The figure shows three views and two pictorial views of one solid part (mm, origin at its lowest corner). Answer the questions. A direction names the side the tool comes from. Coordinates: 2 decimals unless noted, no trailing zeros. Loops run counter-clockwise (first coordinate to the right, second up) from the corner with the lowest first, then second, coordinate; pieces in that order, holes last. Notation, with made-up numbers: M 55.25,47 L 111.25,47 A23 ccw 111.25,60 Z; hole C 77,-25 d4. An arc over 180 degrees is marked long. Return JSON: item names as keys, results as strings. Group by question number.
1. Straight lines are drawn through the part: L1, parallel to X at y = 7.5, z = 41.5; L2, parallel to Z at x = 100, y = 7.7. For each, find the intervals that lie inside material, in ascending order. Write a range as from..to.
2. Section B-B (x = 100) is taken. Write down the section's boundary in (y, z), then the cut area to 3 significant figures.
3. Which of the six approach directions +Z, -Z, +X, -X, +Y, -Y give full straight-line access (tool end or side, diameter ignored) to the marked faces 3 and 4?
4. Section A-A (x = 55) is taken. Write down the section's boundary in (y, z), then the cut area to 3 significant figures.
5. Section D-D (z = 100) is taken. Write down the section's boundary in (x, y).
6. The mould has two halves that part along X. Classify the marked faces 1 and 2: pulls with the +X half, pulls with the -X half, needs draft (parallel to the pull), parting line crosses it, or undercut.
7. Section C-C (y = 8.75) is taken. Write down the section's boundary in (x, z), then the cut area to 3 significant figures.
8. Given P1, Ø4, axis at x = 10, z = 55, coming from the -Y side; P2, Ø1.5, axis at x = 41, z = 75, coming from the -Y side; P3, Ø6, axis at y = 5, z = 16.5, coming from the +X side; P4, Ø5, axis at x = 39, y = 6.5, coming from the -Z side, each flat-ended and moving along its own axis, determine where each tip first touches the part or whether it passes through.
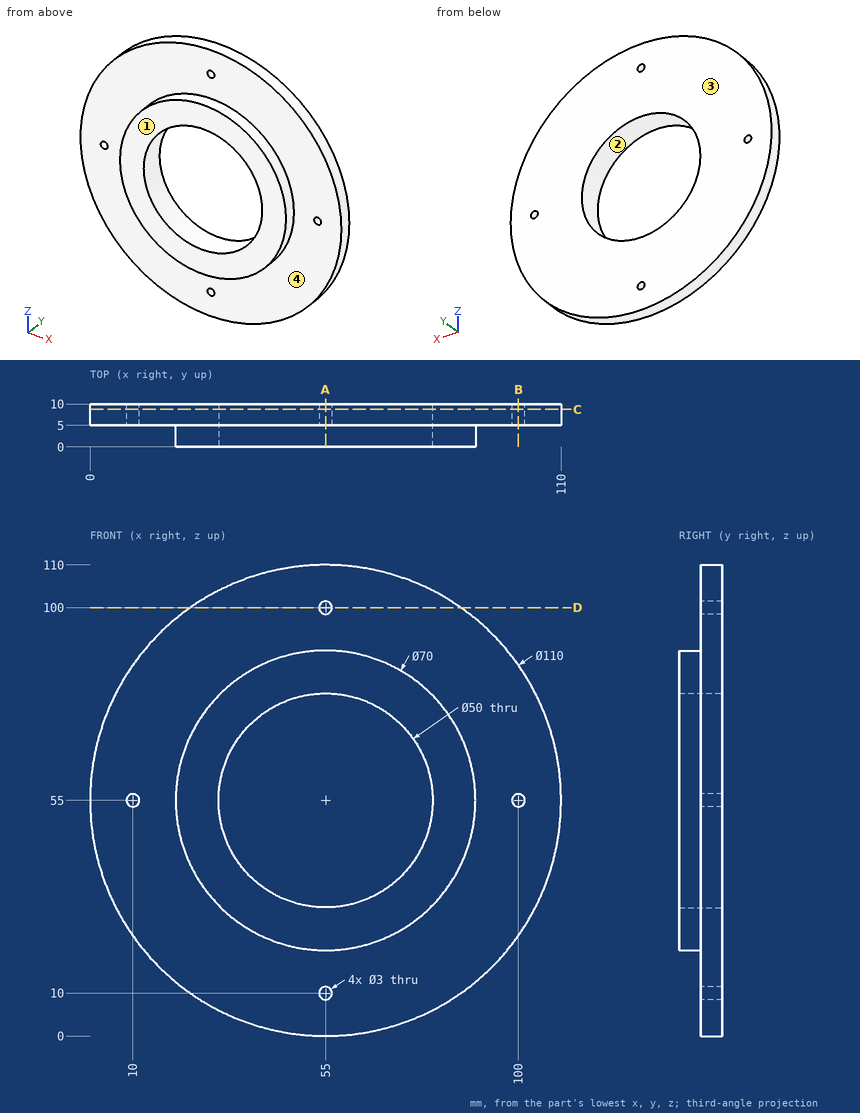
Worked out:
{
 "1": {"L1": "1.68..33.96, 76.04..108.32", "L2": "23.38..53.5, 56.5..86.62"},
 "2": {"outline": "M 5,23.38 L 10,23.38 L 10,53.5 L 5,53.5 Z; M 5,56.5 L 10,56.5 L 10,86.62 L 5,86.62 Z", "area": "301 mm^2"},
 "3": {"face 3": "+Z, -Z, +X, -X, +Y", "face 4": "-Y"},
 "4": {"outline": "M 0,20 L 5,20 L 5,11.5 L 10,11.5 L 10,30 L 0,30 Z; M 0,80 L 10,80 L 10,98.5 L 5,98.5 L 5,90 L 0,90 Z; M 5,0 L 10,0 L 10,8.5 L 5,8.5 Z; M 5,101.5 L 10,101.5 L 10,110 L 5,110 Z", "area": "370 mm^2"},
 "5": {"outline": "M 23.38,5 L 53.5,5 L 53.5,10 L 23.38,10 Z; M 56.5,5 L 86.62,5 L 86.62,10 L 56.5,10 Z"},
 "6": {"face 1": "needs draft", "face 2": "undercut"},
 "7": {"outline": "C 55,55 d110; hole C 10,55 d3; hole C 55,55 d50; hole C 55,10 d3; hole C 55,100 d3; hole C 100,55 d3", "area": "7,510 mm^2"},
 "8": {"P1": "y = 5", "P2": "y = 0", "P3": "x = 97.01", "P4": "z = 1.68"}
}
